from build123d import *

# Parameters (mm, degrees)
SKETCH1_R                 = 9.1
MAIN_DEPTH                = 32
SKETCH2_R                 = 1.35
FIXHOLEMOTORS_DEPTH       = 33
HOLECIRCULARPATTERN_COUNT = 4
SKETCH3_R                 = 15.3
MOTORMAINHOLE_DEPTH       = 27
SKETCH4_W                 = 40
SKETCH4_H                 = 20
CUT_EXTRUDE3_DEPTH        = 27
SKETCH5_R                 = 3.25
HEADSCREWHOLE_DEPTH       = 2
SKETCH6_W                 = 20.2
SKETCH6_H                 = 10.2
WHEELCUT_DEPTH            = 10
SKETCH7_W                 = 20.2
SKETCH7_H                 = 10.2
SKETCH7_R                 = 1.6
BOSS_EXTRUDE2_DEPTH       = 2
FILLET1_R                 = 10
FILLET2_R                 = 10


with BuildPart() as part:
    # Sketch1 → Main (new body)
    with BuildSketch(Plane.XY):
        with BuildLine():
            Line((-5.1, -18), (-1.45, -18))
            Line((-1.45, -18), (-1.45, -19))
            Line((-1.45, -19), (1.45, -19))
            Line((1.45, -19), (1.45, -18))
            Line((1.45, -18), (5.1, -18))
            Line((5.1, -18), (5.1, -21.65))
            Line((5.1, -21.65), (4.1, -21.65))
            Line((4.1, -21.65), (4.1, -24.55))
            Line((4.1, -24.55), (5.1, -24.55))
            Line((5.1, -24.55), (5.1, -28.2))
            Line((5.1, -28.2), (10.1, -28.2))
            Line((10.1, -28.2), (10.1, -18))
            Line((10.1, -18), (20, 0))
            ThreePointArc((20, 0), (0, 20), (-20, 0))
            Line((-20, 0), (-10.1, -18))
            Line((-10.1, -18), (-10.1, -28.2))
            Line((-10.1, -28.2), (-5.1, -28.2))
            Line((-5.1, -28.2), (-5.1, -24.55))
            Line((-5.1, -24.55), (-4.1, -24.55))
            Line((-4.1, -24.55), (-4.1, -21.65))
            Line((-4.1, -21.65), (-5.1, -21.65))
            Line((-5.1, -21.65), (-5.1, -18))
        make_face()
        Circle(SKETCH1_R, mode=Mode.SUBTRACT)
    extrude(amount=MAIN_DEPTH)

    # Sketch2 → FixHoleMotors (cut, through all)
    with BuildSketch(Plane.XY.offset(32)):
        with Locations((0, 13)):
            Circle(SKETCH2_R)
    fixholemotors = extrude(amount=-FIXHOLEMOTORS_DEPTH, mode=Mode.SUBTRACT)

    # HoleCircularPattern: FixHoleMotors ×4 about axis
    holecircularpattern_axis = Axis((0, 0, 0), (0, 0, 1))
    for i in range(1, HOLECIRCULARPATTERN_COUNT):
        add(fixholemotors.rotate(holecircularpattern_axis, i * 360 / HOLECIRCULARPATTERN_COUNT), mode=Mode.SUBTRACT)

    # Sketch3 → MotorMainHole (cut)
    with BuildSketch(Plane.XY):
        Circle(SKETCH3_R)
    extrude(amount=MOTORMAINHOLE_DEPTH, mode=Mode.SUBTRACT)

    # Sketch4 → Cut-Extrude3 (cut)
    with BuildSketch(Plane(origin=(0, 0, 0), x_dir=(-1, 0, 0), z_dir=(0, 0, -1))):
        with Locations((0, 10)):
            Rectangle(SKETCH4_W, SKETCH4_H)
    extrude(amount=-CUT_EXTRUDE3_DEPTH, mode=Mode.SUBTRACT)

    # Sketch5 → HeadScrewHole (cut)
    with BuildSketch(Plane.XY.offset(32)):
        with Locations((0, 13)):
            Circle(SKETCH5_R)
        with Locations((13, 0)):
            Circle(SKETCH5_R)
        with Locations((0, -13)):
            Circle(SKETCH5_R)
        with Locations((-13, 0)):
            Circle(SKETCH5_R)
    extrude(amount=-HEADSCREWHOLE_DEPTH, mode=Mode.SUBTRACT)

    # Sketch6 → WheelCut (cut)
    with BuildSketch(Plane.XY.offset(32)):
        with Locations((0, -23.1)):
            Rectangle(SKETCH6_W, SKETCH6_H)
    extrude(amount=-WHEELCUT_DEPTH, mode=Mode.SUBTRACT)

    # Sketch7 → Boss-Extrude2 (add)
    with BuildSketch(Plane.XY.offset(22)):
        with Locations((0, -23.1)):
            Rectangle(SKETCH7_W, SKETCH7_H)
        with Locations((0, -23.15)):
            Circle(SKETCH7_R, mode=Mode.SUBTRACT)
    extrude(amount=BOSS_EXTRUDE2_DEPTH)

    # Fillet1
    fillet1_edges = [part.edges().sort_by_distance(p)[0] for p in [
        (-10.1, -18, 28),
        (10.1, -18, 28),
    ]]
    fillet(fillet1_edges, radius=FILLET1_R)

    # Fillet2
    fillet2_edges = [part.edges().sort_by_distance(p)[0] for p in [
        (-10.1, -18, 12),
        (10.1, -18, 12),
    ]]
    fillet(fillet2_edges, radius=FILLET2_R)


solid = part.part
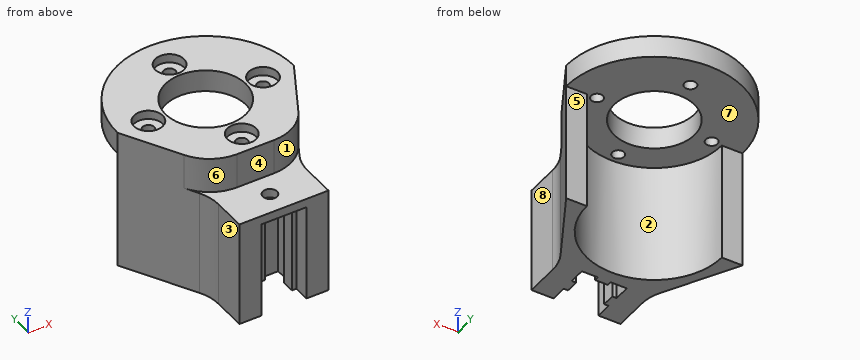
Design review of the part built by this model. Coordinates are the model's own, in mm. Face numbers are marked on the shaded views. A direction names the side the tool comes from. Round coordinates to 2 decimals unless told otherwise and drop trailing zeros. Write each loop counter-clockwise with the first axis right and the second up, starting at its lowest first coordinate (ties: lowest second). Pieces come first, ordered by that corner, then holes.
Item 1: Consider section C-C on z = 15. Give the boundary of the cut face in (x, y).
Item 2: For pin 1 Ø12 at (x, y) = (10.5, 13.5) entering from -Z; pin 2 Ø4 at (y, z) = (-24.5, 12) entering from -X; pin 3 Ø6 at (y, z) = (-5, 21.5) entering from +X; pin 4 Ø16.5 at (x, y) = (0, 0) entering from -Z, all flat-tipped, find the tip position at first contact; note any pin that passes through.
Item 3: Wall thickness on L1, parallel to Y at x = 0, z = 31.15; L2, parallel to X at y = 0, z = 28.95; L3, parallel to Y at x = 0, z = 28.2: over which ranges is each line inside the solid? List them lowest first.
Item 4: Consider section A-A on y = -23.15. Give the boundary of the cut face in (x, z).
Item 5: Draft analysis for pull direction X (two halves, no side actions). For the marked faces 6, 7 and 8, state which applies: released by +X, released by -X, zero draft, split by the parting line, or undercut.
Item 6: Consider section D-D on x = -8. Give the boundary of the cut face in (y, z).
Item 7: For the marked faces 1, 2, 3, 4 and 5, list the 3-axis set-ups (+Z, -Z, +X, -X, +Y, -Y) from which the entire face can be reached by the end or side of a thin tool; tool diameter is ignored.
Item 8: Consider section B-B on x = 0. Count the separate pieces of the cut face and the enclosed holes in it, and give its area (3 significant figures).
Check values:
1. outline: (-20, 0) - (-11.34, -15.75) arc R10 cw to (-10.1, -20.57) - (-10.1, -28.2) - (-5.1, -28.2) - (-5.1, -24.55) - (-4.1, -24.55) - (-4.1, -21.65) - (-5.1, -21.65) - (-5.1, -18) - (-1.45, -18) - (-1.45, -19) - (1.45, -19) - (1.45, -18) - (5.1, -18) - (5.1, -21.65) - (4.1, -21.65) - (4.1, -24.55) - (5.1, -24.55) - (5.1, -28.2) - (10.1, -28.2) - (10.1, -20.57) arc R10 cw to (11.34, -15.75) - (20, 0) - (15.3, 0) arc R15.3 cw to (-15.3, 0) - close
2. pin 1: stops at z = 27
2. pin 2: stops at x = -10.1
2. pin 3: stops at x = 18.9
2. pin 4: passes through
3. L1: y = -18 to -16.25, -9.75 to -9.1, 9.1 to 9.75, 16.25 to 20
3. L2: x = -20 to -14.35, -11.65 to -9.1, 9.1 to 11.65, 14.35 to 20
3. L3: y = -18 to -14.35, -11.65 to -9.1, 9.1 to 11.65, 14.35 to 20
4. outline: (-10.1, 0) - (-4.1, 0) - (-4.1, 22) - (-1.6, 22) - (-1.6, 24) - (-10.1, 24) - close; (1.6, 22) - (4.1, 22) - (4.1, 0) - (10.1, 0) - (10.1, 24) - (1.6, 24) - close
5. face 6: released by -X
5. face 7: undercut
5. face 8: released by +X
6. outline: (-28.2, 0) - (-13.04, 0) - (-13.04, 27) - (-4.34, 27) - (-4.34, 32) - (-17.24, 32) - (-17.24, 24) - (-28.2, 24) - close; (4.34, 27) - (18.33, 27) - (18.33, 32) - (4.34, 32) - close
7. face 1: +Z, +X, -Y
7. face 2: -Z, +Y
7. face 3: +Z, -Z, -X, -Y
7. face 4: +Z, +X, -X, -Y
7. face 5: -Z, +X, -X, +Y
8. separate pieces: 5
8. enclosed holes: 0
8. area: 166 mm2
